Work out the finished part from the listing and answer in its coordinate system (mm). A direction names the side the tool comes from. Round coordinates to 2 decimals unless told otherwise and drop trailing zeros. Write each loop counter-clockwise with the first axis right and the second up, starting at its lowest first coordinate (ties: lowest second). Pieces come first, ordered by that corner, then holes. Notation, with made-up numbers: (0.5, -5) -> (49.5, -5) arc R5 ccw to (49.5, -1) -> close; hole circle Ø4 at (75, 41.25). An arc over 180 degrees is marked (long way). One line per question, with ' | ' between items. Start each with the question number.
Autodesk Inventor part; units mm, degrees
ref_plane "YZ Plane" through (0, 0, 0) normal (1, 0, 0) x (0, 1, 0)
ref_plane "XZ Plane" through (0, 0, 0) normal (0, 1, 0) x (-1, 0, 0)
ref_plane "XY Plane" through (0, 0, 0) normal (0, 0, 1) x (1, 0, 0)
sketch "Sketch1" plane through (0, 0, 0) normal (0, 0, 1) x (1, 0, 0)
  line L0 (0, 102.997) -> (0, 0)
  line L1 (0, 0) -> (142, 0)
  line L2 (142, 0) -> (142, 102.997)
  line L3 (142, 102.997) -> (128, 102.997)
  line L4 (128, 102.997) -> (128, 16.637)
  line L5 (128, 16.637) -> (14, 16.637)
  line L6 (14, 16.637) -> (14, 102.997)
  line L7 (14, 102.997) -> (0, 102.997)
  circle A0 centre (7, 96.997) radius 2.2
  circle A1 centre (135, 96.997) radius 2.2
  circle A2 centre (7, 8.997) radius 2.2
  circle A3 centre (135, 8.997) radius 2.2
  line L8 (14, 102.997) -> (128, 102.997)
  line L9 (28, 102.997) -> (114, 102.997)
  line L10 (114, 0) -> (28, 0)
  line L11 (135, 96.997) -> (135, 8.997) construction
  line L12 (7, 96.997) -> (7, 8.997) construction
  point P0 (71, 102.997)
  dimension "d0" = 102.997
  dimension "d3" = 14
  dimension "d4" = 86.36
  dimension "d44" = 4.4
  dimension "d45" = 4.4
  dimension "d46" = 128
  dimension "d47" = 7
  dimension "d48" = 14
  dimension "d49" = 7
  dimension "d50" = 114
  dimension "d51" = 4.4
  dimension "d52" = 4.4
  dimension "d53" = 88
  dimension "d54" = 88
  dimension "d55" = 6
  dimension "d56" = 6
  dimension "d84" = 128
extrude "Extrusion1" add sketch "Sketch1" along normal blind 26 contours L7 L6 L5 L4 L3 L2 L1 L0
sketch "Sketch5" plane through (14, 16.637, 0) normal (0, 1, 0) x (1, 0, 0)
  line L0 (0, 0) -> (0, -26)
  line L1 (114, 0) -> (114, -26)
  line L2 (114, 0) -> (0, 0) construction
  line L3 (57, 0) -> (57, -26) construction
  line L4 (0, -13) -> (114, -13) construction
  circle A0 centre (28.425, -13) radius 2.75
  circle A1 centre (85.575, -13) radius 2.75
  point P0 (-14, 0)
  dimension "d57" = 5.5
  dimension "d58" = 28.575
extrude "Extrusion2" cut sketch "Sketch5" against normal blind 26
equation "\"d3\" = d48"
equation "\"d44\" = d45"
equation "\"d47\" = 0.5 * d48"
equation "\"d49\" = 0.5 * d3"
equation "\"d51\" = d44"
equation "\"d52\" = d45"
equation "\"d54\" = d53"
equation "\"d56\" = d55"
properties part number "Vertical Electronics Spacer"
(1) For faces 5 (the flat face through (135, 102.997, 13)), 6 (the flat face through (14, 59, 13)), determine the directions among +Z, -Z, +X, -X, +Y, -Y from which every point of the face is accessible in a straight line to the end or side of a thin tool.
(2) A cutting plane is placed at B-B, the plane x = 135. Determine the outline of the cut face in (y, z).
(3) Given pin 1 Ø7 at (x, y) = (135, 8.997) entering from +Z; pin 2 Ø4 at (x, y) = (135, 96.997) entering from +Z; pin 3 Ø1.5 at (x, z) = (18.5, 15) entering from +Y, each flat-ended and moving along its own axis, determine where each tip first touches the part or whether it passes through.
(4) Consider L1, parallel to Y at x = 135, z = 12.5; L2, parallel to X at y = 54.5, z = 17.5; L3, parallel to Y at x = 23, z = 4.25. Determine where each line is inside the solid, lowest interval first.
(5) The mould has two halves that part along Z. Classify faces 1 (the cylindrical face through (96.828, 8.435, 12.879)), 2 (the flat face through (71, 10, 26)), 3 (the flat face through (7, 102.997, 13)), 4 (the cylindrical face through (45.048, 8.435, 12.174)): +Z half, -Z half, draft (parallel to the pull), parting line (faces both ways), or undercut.
(6) A cutting plane is placed at A-A, the plane y = 72.5. Determine the outline of the cut face in (x, z).
(7) A cutting plane is placed at C-C, the plane z = 13. Determine the outline of the cut face in (x, y) (3 decimals).
(8) A cutting plane is placed at D-D, the plane z = 3.5. Determine the outline of the cut face in (x, y), then the cut area to 3 significant figures.
Returned:
1) face 5: +Z, -Z, +X, -X, +Y | face 6: +Z, -Z, +Y
2) outline: (0, 0) -> (6.8, 0) -> (6.8, 26) -> (0, 26) -> close; (11.2, 0) -> (94.8, 0) -> (94.8, 26) -> (11.2, 26) -> close; (99.2, 0) -> (103, 0) -> (103, 26) -> (99.2, 26) -> close
3) pin 1: z = 26 | pin 2: through | pin 3: y = 16.64
4) L1: 0 to 6.8, 11.2 to 94.8, 99.2 to 103 | L2: 0 to 14, 128 to 142 | L3: 0 to 16.64
5) face 1: undercut | face 2: +Z half | face 3: draft | face 4: undercut
6) outline: (0, 0) -> (14, 0) -> (14, 26) -> (0, 26) -> close; (128, 0) -> (142, 0) -> (142, 26) -> (128, 26) -> close
7) outline: (0, 0) -> (39.675, 0) -> (39.675, 16.637) -> (14, 16.637) -> (14, 102.997) -> (0, 102.997) -> close; (45.175, 0) -> (96.825, 0) -> (96.825, 16.637) -> (45.175, 16.637) -> close; (102.325, 0) -> (142, 0) -> (142, 102.997) -> (128, 102.997) -> (128, 16.637) -> (102.325, 16.637) -> close; hole circle Ø4.4 at (7, 8.997); hole circle Ø4.4 at (7, 96.997); hole circle Ø4.4 at (135, 8.997); hole circle Ø4.4 at (135, 96.997)
8) outline: (0, 0) -> (142, 0) -> (142, 103) -> (128, 103) -> (128, 16.64) -> (14, 16.64) -> (14, 103) -> (0, 103) -> close; hole circle Ø4.4 at (7, 9); hole circle Ø4.4 at (7, 97); hole circle Ø4.4 at (135, 9); hole circle Ø4.4 at (135, 97) | area: 4,720 mm2
